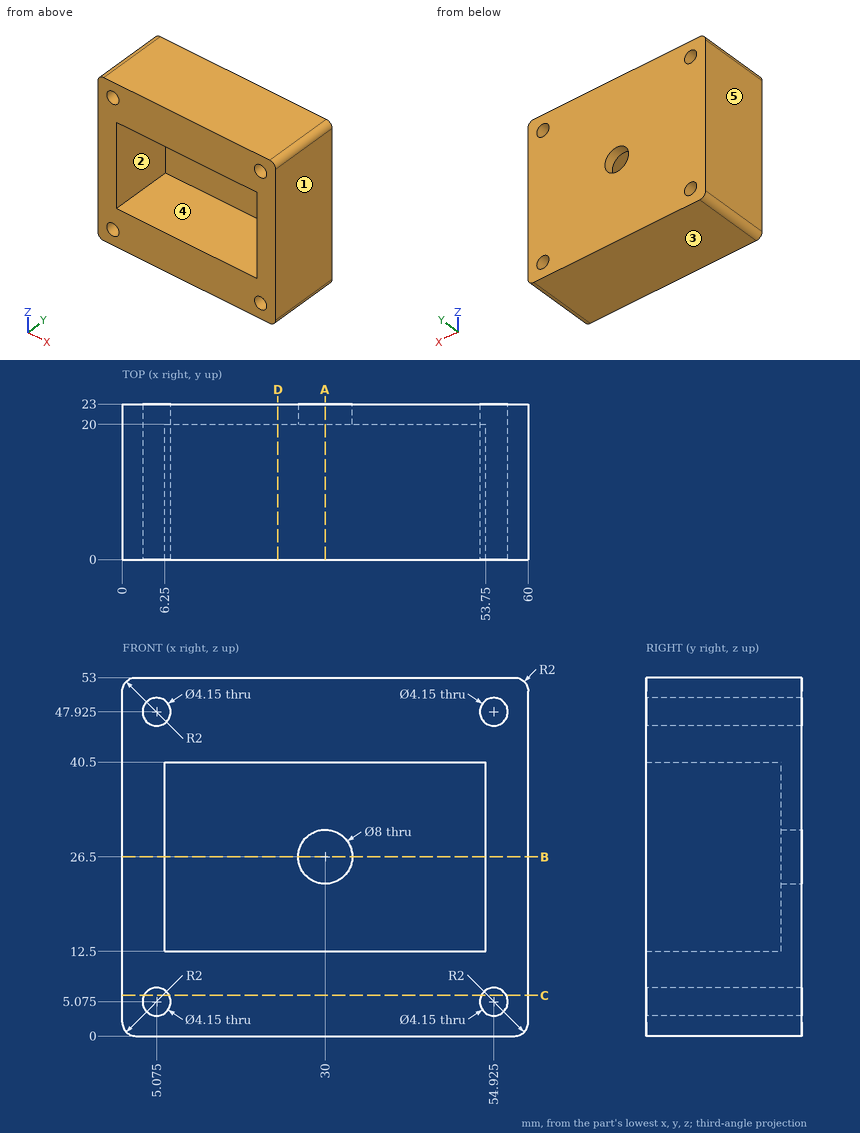
Drawing for the job (mm, zero at the part's lowest x, y, z). A direction names the side the tool comes from. Round coordinates to 2 decimals unless told otherwise and drop trailing zeros. Write each loop counter-clockwise with the first axis right and the second up, starting at its lowest first coordinate (ties: lowest second). Pieces come first, ordered by that corner, then holes. Notation, with made-up numbers: (83.25, 45.5) - (89.25, 45.5) arc R8 cw to (89.25, 58.5) - close; hole circle Ø3 at (-35, -12.75). An arc over 180 degrees is marked (long way). Return JSON: item names as keys, results as strings. Group by question number.
Item 1: Mould opens along X. For the marked faces 3, 4 and 5 say: +X half, -X half, draft (parallel to the pull), parting line (faces both ways), or undercut.
Item 2: Band-saw the part on A-A on x = 30. List the corners of the cut face in (y, z), plus the area to 3 significant figures.
Item 3: Probe probe 1 along X at (y, z) = (10.5, 48); probe 2 along X at (y, z) = (2, 34.5); probe 3 along Z at (x, y) = (22.5, 10.5). List the from-to ranges inside material, lowest first.
Item 4: Band-saw the part on D-D on x = 23. List the corners of the cut face in (y, z).
Item 5: Band-saw the part on B-B on z = 26.5. List the corners of the cut face in (x, y).
Item 6: Flat gauge pins, fed straight in: pin 1 Ø6.5 at (x, z) = (54.925, 5.075) entering from -Y; pin 2 Ø6.5 at (x, z) = (30, 26.5) entering from -Y. Where does each tip first touch, or does it go through?
Item 7: 3-axis set-ups, long thin cutter, end or side, ignore diameter. For the marked faces 1 and 2: which of +Z, -Z, +X, -X, +Y, -Y reach the whole face in a straight line?
Item 8: Band-saw the part on C-C on z = 6. List the corners of the cut face in (x, y), plus the area to 3 significant figures.
Resolved:
{
 "1": {"face 3": "draft", "face 4": "undercut", "face 5": "-X half"},
 "2": {"outline": "(0, 0) - (23, 0) - (23, 22.5) - (20, 22.5) - (20, 12.5) - (0, 12.5) - close; (0, 40.5) - (20, 40.5) - (20, 30.5) - (23, 30.5) - (23, 53) - (0, 53) - close", "area": "635 mm²"},
 "3": {"probe 1": "x = 0 to 3, 7.15 to 52.85, 57 to 60", "probe 2": "x = 0 to 6.25, 53.75 to 60", "probe 3": "z = 0 to 12.5, 40.5 to 53"},
 "4": {"outline": "(0, 0) - (23, 0) - (23, 53) - (0, 53) - (0, 40.5) - (20, 40.5) - (20, 12.5) - (0, 12.5) - close"},
 "5": {"outline": "(0, 0) - (6.25, 0) - (6.25, 20) - (26, 20) - (26, 23) - (0, 23) - close; (34, 20) - (53.75, 20) - (53.75, 0) - (60, 0) - (60, 23) - (34, 23) - close"},
 "6": {"pin 1": "stops at y = 0", "pin 2": "passes through"},
 "7": {"face 1": "+Z, -Z, +X, +Y, -Y", "face 2": "-Y"},
 "8": {"outline": "(0, 0) - (3.22, 0) - (3.22, 23) - (0, 23) - close; (6.93, 0) - (53.07, 0) - (53.07, 23) - (6.93, 23) - close; (56.78, 0) - (60, 0) - (60, 23) - (56.78, 23) - close", "area": "1,210 mm²"}
}
